Check sheet for the modelled part. Datum: model origin and axes. Units: mm. A direction names the side the tool comes from. Give positions to 0.01 mm unless a question says otherwise; leave off trailing zeros. Write each loop counter-clockwise with the first axis right and the second up, starting at its lowest first coordinate (ties: lowest second). Pieces come first, ordered by that corner, then holes. Notation, with made-up numbers: M 30.5,34 L 80.5,34 A15 cw 80.5,41 Z; hole C 2,50.5 d6. An arc over 180 degrees is marked long. Use CSV: the item, a comma, the result in double quotes. Start each with the question number.
1. Access from +Z, -Z, +X, -X, +Y, -Y to the whole of each face (thin tool, end or side, straight path). Record for faces 4 (the face through (-176.486, 5.07, 35.703)), 5 (the face through (378.945, 5.07, 330.979)).
2. Depth check by flat-ended pin: P1, Ø1.5, axis at x = -281.5, z = 267, coming from the -Y side; P2, Ø2, axis at x = 197, y = 2.5, coming from the +Z side; P3, Ø5, axis at y = 6.5, z = -148.5, coming from the +X side; P4, Ø3, axis at x = 286, y = 4, coming from the -Z side. Enter the tip coordinate at first touch or a pass-through.
3. Cross-section at B-B, the plane y = 4. Enter the section's corners in (x, z).
4. Cross-section at D-D, the plane z = -123. Enter the section's corners in (x, y), and give its area (3 significant figures).
5. Mould release check, pull along X, two halves, no side actions. Record for faces 1 (the face through (236.521, 4.93, 331.445)), 2 (the face through (198.203, 5.07, -46.014)), 3 (the face through (-92, 0, -80)): +X half, -X half, draft (parallel to the pull), parting line (faces both ways), or undercut.
6. Scan lines: line 1 (X direction, y = 2.5, z = 105); line 2 (X direction, y = 6, z = -70); line 3 (Z direction, x = 255, y = 4). Record each from-to range of solid material in increasing order.
7. Cross-section at A-A, the plane z = 200. Enter the section's corners in (x, y).
8. Cross-section at C-C, the plane x = 328.5. Enter the section's corners in (y, z), and give its area (3 significant figures).
from build123d import *

# Parameters (mm, degrees)
ESBO_O1_W                = 775
ESBO_O1_H                = 680
RESSALTO_EXTRUS_O1_DEPTH = 10
CORTE_EXTRUS_O1_DEPTH    = 516.612499848
FILETE1_R                = 30


with BuildPart() as part:
    # Esboço1 → Ressalto-extrusão1 (new body)
    with BuildSketch(Plane(origin=(0, 0, 0), x_dir=(1, 0, 0), z_dir=(0, 1, 0))):
        Rectangle(ESBO_O1_W, ESBO_O1_H)
    extrude(amount=RESSALTO_EXTRUS_O1_DEPTH)

    # Esboço2 → Corte-extrusão1 (cut, through all)
    with BuildSketch(Plane(origin=(0, 10, 0), x_dir=(1, 0, 0), z_dir=(0, 1, 0))):
        with BuildLine():
            Line((387.5, 340), (192.5, 340))
            Line((192.5, 340), (192.5, 60))
            ThreePointArc((192.5, 60), (198.357864376, 45.857864376), (212.5, 40))
            Line((212.5, 40), (387.5, 40))
            Line((387.5, 40), (387.5, 340))
        make_face()
        with BuildLine():
            Line((-182.5, -340), (227.5, -340))
            Line((227.5, -340), (227.5, -50))
            ThreePointArc((227.5, -50), (221.642135624, -35.857864376), (207.5, -30))
            Line((207.5, -30), (-162.5, -30))
            ThreePointArc((-162.5, -30), (-176.642135624, -35.857864376), (-182.5, -50))
            Line((-182.5, -50), (-182.5, -340))
        make_face()
    extrude(amount=-CORTE_EXTRUS_O1_DEPTH, mode=Mode.SUBTRACT)

    # Filete1
    filete1_edges = [part.edges().sort_by_distance(p)[0] for p in [
        (-182.5, 5, 340),
        (227.5, 5, 340),
        (387.5, 5, 340),
        (-387.5, 5, 340),
    ]]
    fillet(filete1_edges, radius=FILETE1_R)


solid = part.part
Worked answers:
1,face 4,"+Z, +Y, -Y"
1,face 5,"+Z, +X, +Y, -Y"
2,P1,"stops at y = 0"
2,P2,"stops at z = 30"
2,P3,"stops at x = 192.5"
2,P4,"stops at z = -40"
3,outline,"M -387.5,-340 L 192.5,-340 L 192.5,-60 A20 cw 212.5,-40 L 387.5,-40 L 387.5,310 A30 ccw 357.5,340 L 257.5,340 A30 ccw 227.5,310 L 227.5,50 A20 cw 207.5,30 L -162.5,30 A20 cw -182.5,50 L -182.5,310 A30 ccw -212.5,340 L -357.5,340 A30 ccw -387.5,310 Z"
4,outline,"M -387.5,0 L 192.5,0 L 192.5,10 L -387.5,10 Z"
4,area,"5,800 mm^2"
5,face 1,"undercut"
5,face 2,"+X half"
5,face 3,"draft"
6,line 1,"x = -387.5 to -182.5, 227.5 to 387.5"
6,line 2,"x = -387.5 to 192.5"
6,line 3,"z = -40 to 339.9"
7,outline,"M -387.5,0 L -182.5,0 L -182.5,10 L -387.5,10 Z; M 227.5,0 L 387.5,0 L 387.5,10 L 227.5,10 Z"
8,outline,"M 0,-40 L 10,-40 L 10,340 L 0,340 Z"
8,area,"3,800 mm^2"
